from build123d import *

# Parameters (mm, degrees)
F0_W     = 113.7392967939
F0_H     = 51.4718480408
F1_DEPTH = 32.8
F2_R     = 5
F3_T     = -9
F4_W     = 32.5862057507
F4_H     = 8.9224129915
F5_DEPTH = 38.3
F6_R     = 5
F7_R     = 5.2692974362
F7_R_2   = 5.120837474
F7_R_3   = 5.2226793455
F7_R_4   = 5.2226798643
F8_DEPTH = 15


with BuildPart() as f1:
    # F0 (on Front) → F1 (new body)
    with BuildSketch(Plane.XZ):
        Rectangle(F0_W, F0_H)
    extrude(amount=F1_DEPTH)

    # F2
    f2_edges = [f1.edges().sort_by_distance(p)[0] for p in [
        (56.869648, -16.4, 25.735924),
        (56.869648, -16.4, -25.735924),
        (-56.869648, -16.4, -25.735924),
        (-56.869648, -16.4, 25.735924),
    ]]
    fillet(f2_edges, radius=F2_R)

    # F3
    f3_openings = [f1.faces().sort_by_distance(p)[0] for p in [
        (0, -32.8, 0),
    ]]
    offset(amount=F3_T, openings=f3_openings)

    # F4 (on face) → F5 (cut)
    with BuildSketch(Plane.XY.offset(25.7359240204)):
        with Locations((0, -12.8017254174)):
            Rectangle(F4_W, F4_H)
    extrude(amount=-F5_DEPTH, mode=Mode.SUBTRACT)

    # F6
    f6_edges = [f1.edges().sort_by_distance(p)[0] for p in [
        (47.869648, -20.9, -16.735924),
        (-47.869648, -20.9, -16.735924),
        (-47.869648, -20.9, 16.735924),
        (47.869648, -20.9, 16.735924),
    ]]
    fillet(f6_edges, radius=F6_R)

    # F7 (on face) → F8 (join)
    with BuildSketch(Plane(origin=(0, 0, -25.7359240204), x_dir=(1, 0, 0), z_dir=(0, 0, -1))):
        with Locations((-45.1939664781, 6.4008627087)):
            Circle(F7_R)
        with Locations((-45.7758642733, 26.1853467673)):
            Circle(F7_R_2)
        with Locations((43.8362061977, 6.2068966217)):
            Circle(F7_R_3)
        with Locations((43.8362061977, 25.6034508348)):
            Circle(F7_R_4)
    extrude(amount=F8_DEPTH)


solid = f1.part
Geometry check sheet. Reference: the model listing, model coordinates, mm. A direction names the side the tool comes from. Round coordinates to 2 decimals unless told otherwise and drop trailing zeros. Write each loop counter-clockwise with the first axis right and the second up, starting at its lowest first coordinate (ties: lowest second). Pieces come first, ordered by that corner, then holes.
Item 1: Section check C-C (y = -29.5). Record the boundary of the cut face in (x, z).
Determined:
outline: (-56.87, -20.74) arc R5 ccw to (-51.87, -25.74) - (-49.68, -25.74) - (-49.68, -40.74) - (-41.87, -40.74) - (-41.87, -25.74) - (40.36, -25.74) - (40.36, -40.74) - (47.31, -40.74) - (47.31, -25.74) - (51.87, -25.74) arc R5 ccw to (56.87, -20.74) - (56.87, 20.74) arc R5 ccw to (51.87, 25.74) - (-51.87, 25.74) arc R5 ccw to (-56.87, 20.74) - close; hole (-47.87, -11.74) arc R5 ccw to (-42.87, -16.74) - (42.87, -16.74) arc R5 ccw to (47.87, -11.74) - (47.87, 11.74) arc R5 ccw to (42.87, 16.74) - (-42.87, 16.74) arc R5 ccw to (-47.87, 11.74) - close
Item 2: Mould release check, pull along Z, two halves, no side actions. Record for faces 6 (the face through (-45, -6, -40.736)), 7 (the face through (48.82, -27.17, -33.13)), 8 (the face through (46.444, -21.067, -15.232)): +Z half, -Z half, draft (parallel to the pull), parting line (faces both ways), or undercut.
Determined:
face 6: -Z half
face 7: draft
face 8: undercut
Item 3: Material ranges on line 1 along Y through (x, z) = (2.5, 19.5); line 2 along X through (y, z) = (-31, 11); line 3 along Z through (x, y) = (-35, -13), recorded low to high.
Determined:
line 1: y = -32.8 to -17.26, -8.34 to 0
line 2: x = -56.87 to -47.87, 47.87 to 56.87
line 3: z = -25.74 to -16.74, 16.74 to 25.74
Item 4: Access from +Z, -Z, +X, -X, +Y, -Y to the whole of each face (thin tool, end or side, straight path). Record for faces 1 (the face through (-16.293, -12, 18)), 2 (the face through (-1, -21, -16.736)), 3 (the face through (-50.46, -6.63, -33.13)), 4 (the face through (56.87, -16, 0)), 5 (the face through (55.366, -16.63, -24.31)).
Determined:
face 1: +Z
face 2: -Y
face 3: -Z
face 4: +Z, -Z, +X, +Y, -Y
face 5: -Z, +X, +Y, -Y
Item 5: Section check B-B (z = -7.5). Record the boundary of the cut face in (x, y), plus the area to 3 significant figures.
Determined:
outline: (-56.87, -32.8) - (-47.87, -32.8) - (-47.87, -9) - (-16.29, -9) - (-16.29, -8.34) - (16.29, -8.34) - (16.29, -9) - (47.87, -9) - (47.87, -32.8) - (56.87, -32.8) - (56.87, 0) - (-56.87, 0) - close
area: 1,430 mm2
Item 6: Section check D-D (y = -14). Record the boundary of the cut face in (x, z), plus the area to 3 significant figures.
Determined:
outline: (-56.87, -20.74) arc R5 ccw to (-51.87, -25.74) - (51.87, -25.74) arc R5 ccw to (56.87, -20.74) - (56.87, 20.74) arc R5 ccw to (51.87, 25.74) - (16.29, 25.74) - (16.29, 16.74) - (42.87, 16.74) arc R5 cw to (47.87, 11.74) - (47.87, -11.74) arc R5 cw to (42.87, -16.74) - (-42.87, -16.74) arc R5 cw to (-47.87, -11.74) - (-47.87, 11.74) arc R5 cw to (-42.87, 16.74) - (-16.29, 16.74) - (-16.29, 25.74) - (-51.87, 25.74) arc R5 ccw to (-56.87, 20.74) - close
area: 2,360 mm2
Item 7: Section check A-A (x = 6). Record the boundary of the cut face in (y, z).
Determined:
outline: (-32.8, -25.74) - (0, -25.74) - (0, 25.74) - (-8.34, 25.74) - (-8.34, -12.56) - (-9, -12.56) - (-9, -16.74) - (-32.8, -16.74) - close; (-32.8, 16.74) - (-17.26, 16.74) - (-17.26, 25.74) - (-32.8, 25.74) - close
Item 8: Go/stop test with flat-tipped pins: pin 1 Ø16.5 at (x, z) = (-16, -6.5) entering from -Y; pin 2 Ø7 at (x, y) = (11.5, -17.5) entering from -Z; pin 3 Ø12 at (x, z) = (2.5, -1) entering from -Y. Record where each tip stops, or that it passes through.
Determined:
pin 1: stops at y = -9
pin 2: stops at z = -25.74
pin 3: stops at y = -8.34
